Source: CAD feature listing. Evaluate the final solid. Frame: model axes, mm. A direction names the side the tool comes from. Round coordinates to 2 decimals unless told otherwise and drop trailing zeros. Loops run counter-clockwise (first coordinate to the right, second up) from the corner with the lowest first, then second, coordinate; pieces in that order, holes last. Notation, with made-up numbers: (-26, -13.75) -> (19, -13.75) arc R23 ccw to (19, 22.25) -> close; hole circle Ø1 at (80.5, 30.5). An arc over 180 degrees is marked (long way). Put each result on its own line as item: value. Start each with the question number.
1. Draft query along X for faces 3 (the flat face through (-254, 39, -4)), 4 (the flat face through (-4, 39, -254)), 5 (the flat face through (-3, 0, 3)). Return one class per face: pulls with the +X half, pulls with the -X half, needs draft (parallel to the pull), parting line crosses it, or undercut.
2. Set-up query: faces 1 (the flat face through (228.6, 50, 3)), 2 (the flat face through (254, 39, -4)). Return all of +Z, -Z, +X, -X, +Y, -Y with unobstructed straight access to the full face (end or side cutting, diameter ignored); none if empty.
3. Cut plane B-B (x = 163.5). Return the cut outline in (y, z).
4. Material intervals for L1, parallel to X at y = -19.5, z = -190.5; L2, parallel to Z at x = 190, y = -7; L3, parallel to Z at x = -163, y = 24.5, sorted ascending.
5. Contact query for flat-ended pins moving along their axis: pin 1 (1.3 mm diameter, centred on x = -196.596, z = -182.126, fed in from -Y); pin 2 (2.5 mm diameter, centred on x = -184.596, z = -199.126, fed in from +Y). Output: stop coordinate, or through.
6. Cut plane C-C (y = 11). Return the cut outline in (x, z), then the cut area to 3 significant figures.
7. Cut plane A-A (z = 14). Return the cut outline in (x, y), then the cut area to 3 significant figures.
```python
from build123d import *

# Parameters (mm, degrees)
SKETCH1_W           = 508
SKETCH1_H           = 508
SKETCH1_W_2         = 457.2
SKETCH1_H_2         = 457.2
BOSS_EXTRUDE1_DEPTH = 101.6
SKETCH2_W           = 508
SKETCH2_H           = 508
BOSS_EXTRUDE2_DEPTH = 25.4
SKETCH3_R           = 0.8
SKETCH3_R_2         = 5.08
CUT_EXTRUDE1_DEPTH  = 25.4


with BuildPart() as part:
    # Sketch1 → Boss-Extrude1 (new body)
    with BuildSketch(Plane(origin=(0, 0, 0), x_dir=(1, 0, 0), z_dir=(0, 1, 0))):
        Rectangle(SKETCH1_W, SKETCH1_H)
        Rectangle(SKETCH1_W_2, SKETCH1_H_2, mode=Mode.SUBTRACT)
    extrude(amount=BOSS_EXTRUDE1_DEPTH)

    # Sketch2 → Boss-Extrude2 (add)
    with BuildSketch(Plane.XZ):
        Rectangle(SKETCH2_W, SKETCH2_H)
    extrude(amount=BOSS_EXTRUDE2_DEPTH)

    # Sketch3 → Cut-Extrude1 (cut)
    with BuildSketch(Plane(origin=(0, 0, 0), x_dir=(1, 0, 0), z_dir=(0, 1, 0))):
        with Locations(Location((-196.596, 199.126, 0), (0, 0, 270))):
            Circle(SKETCH3_R)
        with Locations(Location((-184.596, 199.126, 0), (0, 0, 270))):
            Circle(SKETCH3_R)
        with Locations(Location((-190.5, 190.5, 0), (0, 0, 270))):
            Circle(SKETCH3_R_2)
        with Locations(Location((-184.596, 182.126, 0), (0, 0, 270))):
            Circle(SKETCH3_R)
        with Locations(Location((-196.596, 182.126, 0), (0, 0, 270))):
            Circle(SKETCH3_R)
        with Locations(Location((190.5, 190.5, 0), (0, 0, 90))):
            Circle(SKETCH3_R_2)
        with Locations(Location((184.596, 199.126, 0), (0, 0, 90))):
            Circle(SKETCH3_R)
        with Locations(Location((184.596, 182.126, 0), (0, 0, 90))):
            Circle(SKETCH3_R)
        with Locations(Location((196.596, 182.126, 0), (0, 0, 90))):
            Circle(SKETCH3_R)
        with Locations(Location((196.596, 199.126, 0), (0, 0, 90))):
            Circle(SKETCH3_R)
        with Locations(Location((190.5, -190.5, 0), (0, 0, 270))):
            Circle(SKETCH3_R_2)
        with Locations(Location((-190.5, -190.5, 0), (0, 0, 90))):
            Circle(SKETCH3_R_2)
    extrude(amount=-CUT_EXTRUDE1_DEPTH, mode=Mode.SUBTRACT)


solid = part.part
```
Solution:
1. face 3: pulls with the -X half
1. face 4: needs draft
1. face 5: undercut
2. face 1: +Y
2. face 2: +Z, -Z, +X, +Y, -Y
3. outline: (-25.4, -254) -> (101.6, -254) -> (101.6, -228.6) -> (0, -228.6) -> (0, 228.6) -> (101.6, 228.6) -> (101.6, 254) -> (-25.4, 254) -> close
4. L1: x = -254 to -195.58, -185.42 to 185.42, 195.58 to 254
4. L2: z = -254 to -195.56, -185.44 to 185.44, 195.56 to 254
4. L3: z = -254 to -228.6, 228.6 to 254
5. pin 1: passes through
5. pin 2: stops at y = 0
6. outline: (-254, -254) -> (254, -254) -> (254, 254) -> (-254, 254) -> close; hole (-228.6, -228.6) -> (228.6, -228.6) -> (228.6, 228.6) -> (-228.6, 228.6) -> close
6. area: 49,000 mm^2
7. outline: (-254, -25.4) -> (254, -25.4) -> (254, 101.6) -> (228.6, 101.6) -> (228.6, 0) -> (-228.6, 0) -> (-228.6, 101.6) -> (-254, 101.6) -> close
7. area: 18,100 mm^2
